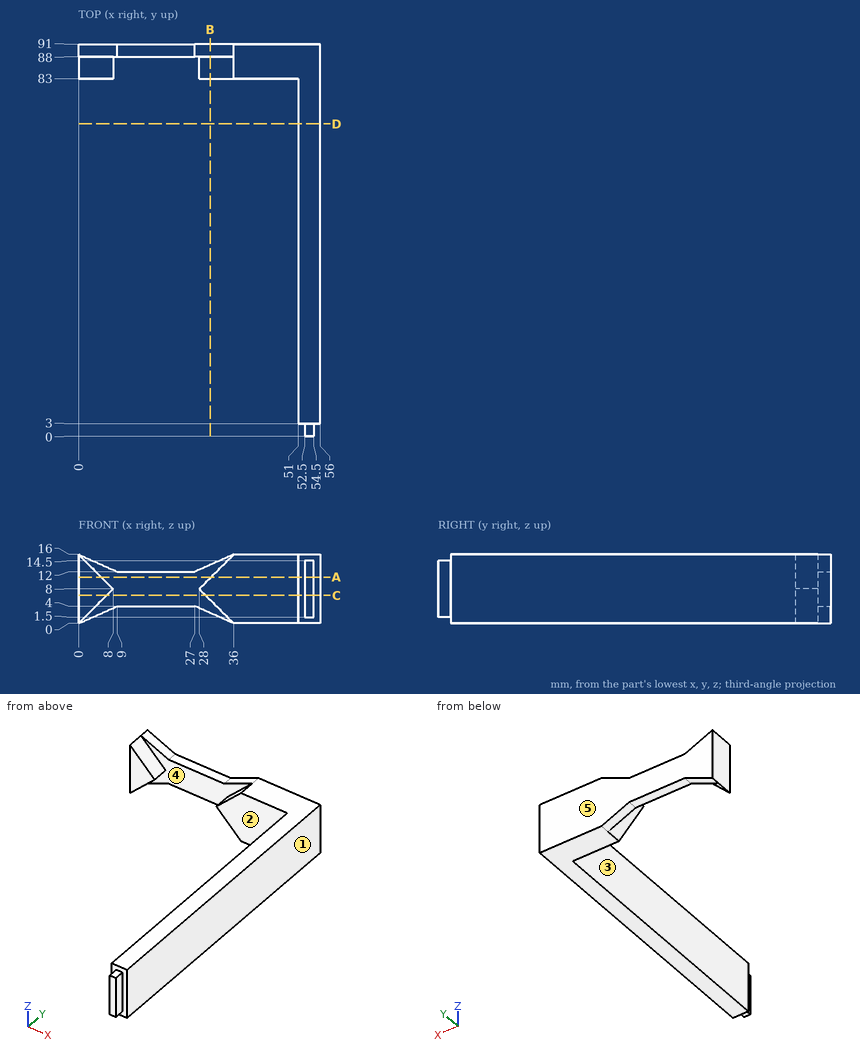
Answer from the drawing. Dimensions are ordinates in mm from the lowest x, y and z of the part. A direction names the side the tool comes from. Round coordinates to 2 decimals unless told otherwise and drop trailing zeros. Write each loop counter-clockwise with the first axis right and the second up, starting at its lowest first coordinate (ties: lowest second). Pieces come first, ordered by that corner, then holes. Notation, with made-up numbers: M 56,50 L 66,50 A28 ccw 66,89 Z; hole C -5.5,35.25 d4. An arc over 180 degrees is marked long. Write each question's results on one line, items separated by ' | '. Start each with the question number.
Item 1: Find section D-D on y = 72.5. Write down the section's boundary in (x, z).
Item 2: Straight lines are drawn through the part: probe 1 along Y at (x, z) = (42, 1.75); probe 2 along X at (y, z) = (7.5, 13); probe 3 along Y at (x, z) = (30, 2.75). For each, find the intervals that lie inside material, in ascending order.
Item 3: Given pin 1 Ø4 at (x, z) = (32.5, 6) entering from -Y; pin 2 Ø3.5 at (x, y) = (13.5, 89.5) entering from -Z; pin 3 Ø2 at (x, z) = (10, 10) entering from -Y; pin 4 Ø1 at (x, z) = (12.5, 2) entering from -Y, each flat-ended and moving along its own axis, determine where each tip first touches the part or whether it passes through.
Item 4: Find section C-C on z = 6.5. Write down the section's boundary in (x, y).
Item 5: Find section A-A on z = 10.75. Write down the section's boundary in (x, y), and give its area (4 significant figures).
Item 6: Find section B-B on x = 30.5. Write down the section's boundary in (y, z).
Item 7: The mould has two halves that part along X. Classify the marked faces 3, 4 and 5: +X half, -X half, draft (parallel to the pull), parting line (faces both ways), or undercut.
Item 8: Which of the six approach directions +Z, -Z, +X, -X, +Y, -Y give full straight-line access (tool end or side, diameter ignored) to the marked faces 1 and 2?
Answer block:
1) outline: M 51,0 L 56,0 L 56,16 L 51,16 Z
2) probe 1: y = 83 to 91 | probe 2: x = 51 to 56 | probe 3: y = 88 to 91
3) pin 1: stops at y = 83 | pin 2: stops at z = 4 | pin 3: stops at y = 88 | pin 4: passes through
4) outline: M 0,83 L 6.5,83 L 6.5,88 L 29.5,88 L 29.5,83 L 51,83 L 51,3 L 52.5,3 L 52.5,0 L 54.5,0 L 54.5,3 L 56,3 L 56,91 L 0,91 Z
5) outline: M 0,83 L 5.25,83 L 5.25,88 L 30.75,88 L 30.75,83 L 51,83 L 51,3 L 52.5,3 L 52.5,0 L 54.5,0 L 54.5,3 L 56,3 L 56,91 L 0,91 Z | area: 726.5 mm²
6) outline: M 83,5.5 L 88,5.5 L 88,2.44 L 91,2.44 L 91,13.56 L 88,13.56 L 88,10.5 L 83,10.5 Z
7) face 3: -X half | face 4: undercut | face 5: draft
8) face 1: +Z, -Z, +X, +Y, -Y | face 2: +Z, -Z, -X, -Y
